```python
from build123d import *

# Parameters (mm, degrees)
BOX004_W        = 80
BOX004_H        = 36.2
BOX004_DEPTH    = 1.6
BOX005_W        = 72
BOX005_H        = 25
BOX005_DEPTH    = 6.7
SKETCH019_R     = 1.5
POCKET002_DEPTH = 5


with BuildPart() as part:
    # Box004 → Box004 (join)
    with BuildSketch(Plane.XY):
        with Locations((40, 18.1)):
            Rectangle(BOX004_W, BOX004_H)
    extrude(amount=BOX004_DEPTH)

    # Box005 → Box005 (join)
    with BuildSketch(Plane(origin=(4, 5.6, 1.6), x_dir=(1, 0, 0), z_dir=(0, 0, 1))):
        with Locations((36, 12.5)):
            Rectangle(BOX005_W, BOX005_H)
    extrude(amount=BOX005_DEPTH)

    # Sketch019 → Pocket002 (cut)
    with BuildSketch(Plane.XY):
        with Locations((2.25, 33.35)):
            Circle(SKETCH019_R)
        with Locations((77.75, 33.35)):
            Circle(SKETCH019_R)
        with Locations((77.75, 2.85)):
            Circle(SKETCH019_R)
        with Locations((2.25, 2.85)):
            Circle(SKETCH019_R)
    extrude(amount=POCKET002_DEPTH, mode=Mode.SUBTRACT)


solid = part.part
```
Can you work these out from the model? Positions are in its coordinate system, mm. A direction names the side the tool comes from. Give positions to 0.01 mm unless a question says otherwise; leave off trailing zeros. Order: outer loops, then holes, each group sorted by start corner. A loop starts at its lowest first (then second) coordinate and runs counter-clockwise, first axis right, second up. Notation, with made-up numbers: M 5,88 L 12,88 A26 cw 12,104 Z; hole C -7.5,63.25 d7. An arc over 180 degrees is marked long. Write item = value, one per line. Start each with the question number.
Q1. Suppose I cut it at D-D (z = 2.75). Write out the boundary of the cut face in (x, y).
Q2. Suppose I cut it at B-B (x = 2.25). Write out the boundary of the cut face in (y, z).
Q3. For faces 5 (the flat face through (4, 18, 5)), 6 (the flat face through (39, 30.6, 5)), 7 (the flat face through (0, 18, 1)), which set-ups out of +Z, -Z, +X, -X, +Y, -Y let a thin tool reach every point of the face, with its end or its side?
Q4. I need wall thicknesses on probe 1 along X at (y, z) = (2.85, 1.1); probe 2 along Y at (x, z) = (2.25, 0.75); probe 3 along X at (y, z) = (26, 5.25). Which ranges of each line are inside material? Lowest first, please. Write a range as [from, to].
Q5. Will these pins go through, and if not, where does the flat tip stop? pin 1 Ø3.5 at (x, z) = (43, 4.5) entering from +Y; pin 2 Ø3 at (y, z) = (20, 4.5) entering from +X; pin 3 Ø3.5 at (x, y) = (2.25, 33.35) entering from +Z.
Q6. Suppose I cut it at C-C (x = 63). Write out the boundary of the cut face in (y, z).
Q7. Suppose I cut it at A-A (y = 2.85). Write out the boundary of the cut face in (x, z), plus the area to 3 significant figures.
Q8. We'd pull the mould along Y, two halves only. Please class faces 1 (the flat face through (39, 5.6, 5)), 2 (the cylindrical face through (1.14, 3.86, 0.79)), 3 (the flat face through (39, 36.2, 1)), 4 (the flat face through (76, 18, 5)): pulls with the +Y half, pulls with the -Y half, needs draft (parallel to the pull), parting line crosses it, or undercut.
Check result:
q1.outline = M 4,5.6 L 76,5.6 L 76,30.6 L 4,30.6 Z
q2.outline = M 0,0 L 1.35,0 L 1.35,1.6 L 0,1.6 Z; M 4.35,0 L 31.85,0 L 31.85,1.6 L 4.35,1.6 Z; M 34.85,0 L 36.2,0 L 36.2,1.6 L 34.85,1.6 Z
q3.face_5 = +Z, -X, +Y, -Y
q3.face_6 = +Z, +X, -X, +Y
q3.face_7 = +Z, -Z, -X, +Y, -Y
q4.probe_1 = [0, 0.75], [3.75, 76.25], [79.25, 80]
q4.probe_2 = [0, 1.35], [4.35, 31.85], [34.85, 36.2]
q4.probe_3 = [4, 76]
q5.pin_1 = 30.6
q5.pin_2 = 76
q5.pin_3 = 1.6
q6.outline = M 0,0 L 36.2,0 L 36.2,1.6 L 30.6,1.6 L 30.6,8.3 L 5.6,8.3 L 5.6,1.6 L 0,1.6 Z
q7.outline = M 0,0 L 0.75,0 L 0.75,1.6 L 0,1.6 Z; M 3.75,0 L 76.25,0 L 76.25,1.6 L 3.75,1.6 Z; M 79.25,0 L 80,0 L 80,1.6 L 79.25,1.6 Z
q7.area = 118 mm2
q8.face_1 = pulls with the -Y half
q8.face_2 = undercut
q8.face_3 = pulls with the +Y half
q8.face_4 = needs draft
